Geometry check sheet. Reference: drawing and pictorial views, mm from the part's lowest x, y, z. Round coordinates to 2 decimals unless told otherwise and drop trailing zeros. Order: outer loops, then holes, each group sorted by start corner. A loop starts at its lowest first (then second) coordinate and runs counter-clockwise, first axis right, second up.
(1) Gauge pin test, flat ends, axial feed: P1, Ø1, axis at x = 15, y = 3.5, coming from the +Z side; P2, Ø3, axis at x = 17.5, y = 3, coming from the -Z side; P3, Ø1, axis at y = 4, z = 64, coming from the +X side. Record the tip position at first contact, or that the pin passes through.
(2) Thickness scan on L1, parallel to Z at x = 42.5, y = 2.75; L2, parallel to Z at x = 73, y = 1; L3, parallel to Z at x = 75.5, y = 5.75. Record the ranges inside material, lowest first.
(3) Cross-section at A-A on z = 55.5. Enter the section's corners in (x, y).
(4) Cross-section at B-B on x = 46.5. Enter the section's corners in (y, z), and give its area (3 significant figures).
(5) Cross-section at D-D on x = 21. Enter the section's corners in (y, z).
(6) Draft check along X on the marked faces 1, 2 and 3. Enter one of: pulls with the +X half, pulls with the -X half, needs draft (parallel to the pull), parting line crosses it, or undercut.
(7) Cross-section at C-C on y = 2.25. Enter the section's corners in (x, z) (3 decimals).
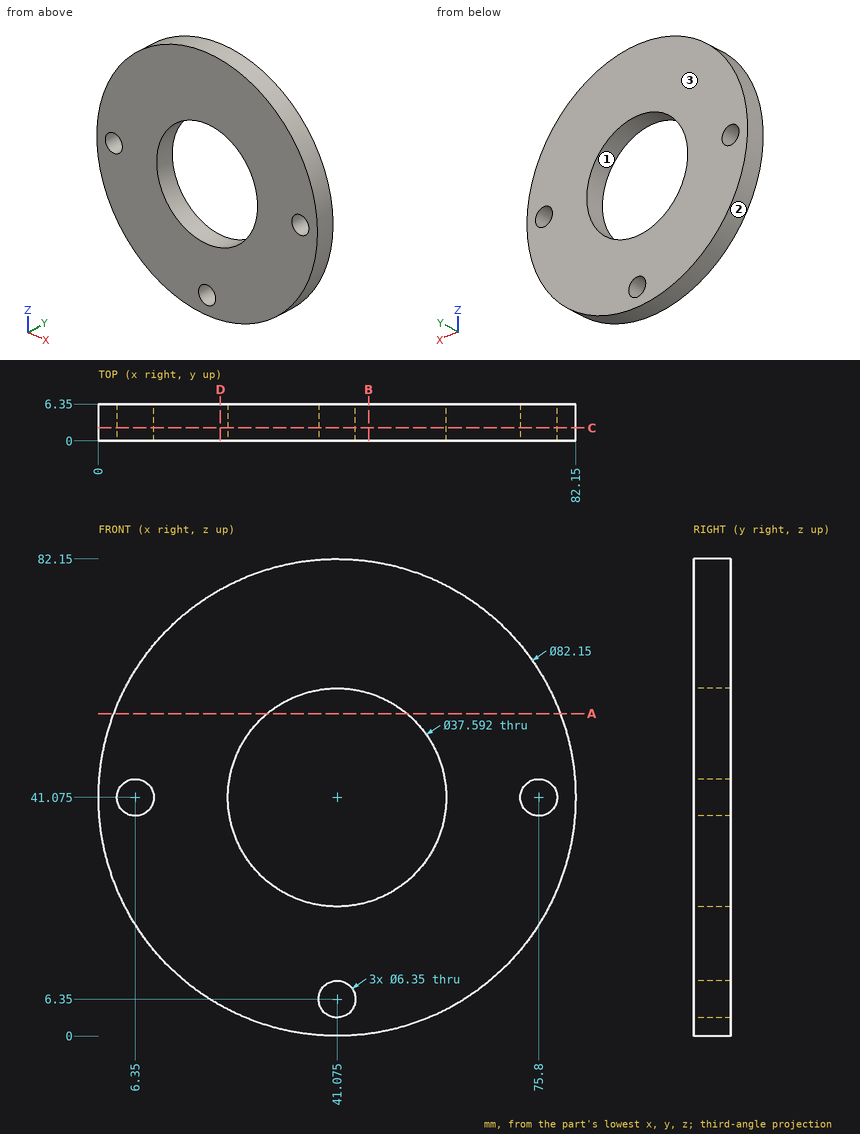
Found:
1. P1: stops at z = 73.22
1. P2: stops at z = 6.44
1. P3: stops at x = 75.49
2. L1: z = 0.02 to 3.51, 9.19 to 22.33, 59.82 to 82.13
2. L2: z = 15.23 to 39.58, 42.57 to 66.92
2. L3: z = 18.67 to 37.91, 44.24 to 63.48
3. outline: (2.62, 0) - (29.02, 0) - (29.02, 6.35) - (2.62, 6.35) - close; (53.13, 0) - (79.53, 0) - (79.53, 6.35) - (53.13, 6.35) - close
4. outline: (0, 0.36) - (6.35, 0.36) - (6.35, 23.08) - (0, 23.08) - close; (0, 59.07) - (6.35, 59.07) - (6.35, 81.79) - (0, 81.79) - close
4. area: 289 mm2
5. outline: (0, 5.24) - (6.35, 5.24) - (6.35, 76.91) - (0, 76.91) - close
6. face 1: undercut
6. face 2: parting line crosses it
6. face 3: needs draft
7. outline: circle Ø82.15 at (41.075, 41.075); hole circle Ø6.35 at (6.35, 41.075); hole circle Ø37.592 at (41.075, 41.075); hole circle Ø6.35 at (41.075, 6.35); hole circle Ø6.35 at (75.8, 41.075)
